Answer from the drawing. Dimensions are ordinates in mm from the lowest x, y and z of the part. A direction names the side the tool comes from. Coordinates: 2 decimals unless noted, no trailing zeros. Order: outer loops, then holes, each group sorted by start corner. A loop starts at its lowest first (then second) coordinate and runs counter-clockwise, first axis right, second up. Notation, with made-up numbers: M 70.25,8.25 L 89.25,8.25 A28 cw 89.25,34.25 Z; hole C -23,-10.75 d2. An arc over 180 degrees is marked long. One line per question, with ' | ' between items. Start each with the question number.
1) Consider probe 1 along Y at (x, z) = (93.5, 10.7); probe 2 along Z at (x, y) = (91, 22.5); probe 3 along Y at (x, z) = (90, 9.5). Determine where each line is inside the solid, lowest interval first.
2) Find section C-C, the plane z = 11. Write down the section's boundary in (x, y).
3) Find section B-B, the plane x = 46. Write down the section's boundary in (y, z).
4) A tool of negligible diameter and unlimited length cuts with its end or side. For the marked faces 1, 2 and 3, from which of +Z, -Z, +X, -X, +Y, -Y can it reach the whole face along a straight path? Write none if from no direction.
5) Find section A-A, the plane x = 6.5. Write down the section's boundary in (y, z).
6) Find section D-D, the plane y = 15.5. Write down the section's boundary in (x, z), plus the area to 3 significant figures.
7) Given P1, Ø3.5, axis at x = 93.5, y = 21, coming from the +Z side; P2, Ø4, axis at x = 69, z = 10.5, coming from the -Y side; P3, Ø5, axis at x = 90, y = 9.5, coming from the -Z side; P4, Ø5, axis at x = 53.5, z = 1.5, coming from the -Y side, each flat-ended and moving along its own axis, determine where each tip first touches the part or whether it passes through.
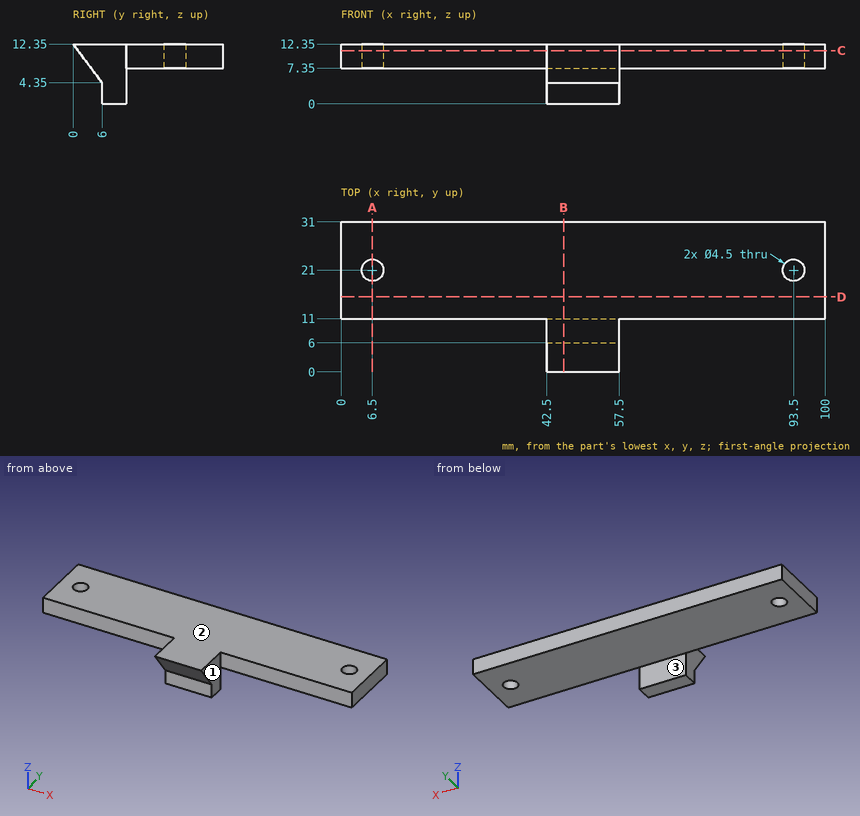
Report:
1) probe 1: y = 11 to 18.75, 23.25 to 31 | probe 2: z = 7.35 to 12.35 | probe 3: y = 11 to 31
2) outline: M 0,11 L 42.5,11 L 42.5,1.01 L 57.5,1.01 L 57.5,11 L 100,11 L 100,31 L 0,31 Z; hole C 6.5,21 d4.5; hole C 93.5,21 d4.5
3) outline: M 0,12.35 L 6,4.35 L 6,0 L 11,0 L 11,7.35 L 31,7.35 L 31,12.35 Z
4) face 1: +Z, -Z, +X, -Y | face 2: +Z, +X, -X, +Y, -Y | face 3: -Z, +X, -X, +Y
5) outline: M 11,7.35 L 18.75,7.35 L 18.75,12.35 L 11,12.35 Z; M 23.25,7.35 L 31,7.35 L 31,12.35 L 23.25,12.35 Z
6) outline: M 0,7.35 L 100,7.35 L 100,12.35 L 0,12.35 Z | area: 500 mm^2
7) P1: passes through | P2: stops at y = 11 | P3: stops at z = 7.35 | P4: stops at y = 6
